Autodesk Inventor part; units mm, degrees
ref_plane "YZ Plane" through (0, 0, 0) normal (1, 0, 0) x (0, 1, 0)
ref_plane "XZ Plane" through (0, 0, 0) normal (0, 1, 0) x (-1, 0, 0)
ref_plane "XY Plane" through (0, 0, 0) normal (0, 0, 1) x (1, 0, 0)
sketch "Sketch1" plane through (0, 0, 0) normal (0, 0, 1) x (1, 0, 0)
  circle A0 centre (0, 0) radius 11
  dimension "d0" = 22
extrude "Extrusion1" add sketch "Sketch1" along normal blind 14
fillet "Fillet1" radius 2 1 edges at (-11, 0, 14)
fillet "Fillet1" radius 4 1 edges at (-11, 0, 0)
hole "Hole1" at (0, 0, 14) direction (0, 0, -1) diameter 13.376 end through all
properties part number "HANDLE CAP" material "Steel, Mild"
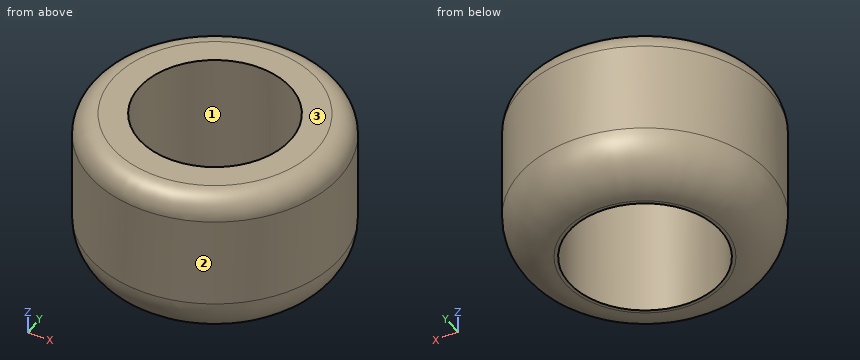
Work out the finished part from the listing and answer in its coordinate system (mm). Face numbers are marked on the shaded views. Round coordinates to 2 decimals unless told otherwise and drop trailing zeros. Write each loop counter-clockwise with the first axis right and the second up, starting at its lowest first coordinate (ties: lowest second). Pieces come first, ordered by that corner, then holes.
1) Consider probe 1 along Y at (x, z) = (0, 6.75); probe 2 along Y at (x, z) = (5.75, 7.75); probe 3 along X at (y, z) = (-2.75, 10.25). Determine where each line is inside the solid, lowest interval first.
2) A cutting plane is placed at C-C on z = 8. Determine the outline of the cut face in (x, y), and give its area (3 significant figures).
3) Determine the mould class of the marked faces 1, 2 and 3 for opening direction Y: pulls with the +Y half, pulls with the -Y half, needs draft (parallel to the pull), parting line crosses it, or undercut.
4) A cutting plane is placed at D-D on z = 3.5. Determine the outline of the cut face in (x, y).
5) Flat-ended cylindrical pins translate along their axes: P1, Ø8, axis at y = -5.5, z = 8, coming from the +X side; P2, Ø4, axis at x = -1, z = 6, coming from the -Y side; P3, Ø6, axis at y = 7, z = 9.5, coming from the -X side; P4, Ø6, axis at y = 5, z = 2, coming from the -X side. Find the tip coordinate at first contact, or state that the pin passes through.
6) A cutting plane is placed at A-A on y = 0. Determine the outline of the cut face in (x, z), and give its area (3 significant figures).
Entries:
1. probe 1: y = -11 to -6.69, 6.69 to 11
1. probe 2: y = -9.38 to -3.42, 3.42 to 9.38
1. probe 3: x = -10.65 to -6.1, 6.1 to 10.65
2. outline: circle Ø22 at (0, 0); hole circle Ø13.38 at (0, 0)
2. area: 240 mm2
3. face 1: undercut
3. face 2: parting line crosses it
3. face 3: needs draft
4. outline: circle Ø21.94 at (0, 0); hole circle Ø13.38 at (0, 0)
5. P1: stops at x = 10.9
5. P2: stops at y = -11
5. P3: stops at x = -10.25
5. P4: stops at x = -10.7
6. outline: (-11, 4) arc R4 ccw to (-7, 0) - (-6.69, 0) - (-6.69, 14) - (-9, 14) arc R2 ccw to (-11, 12) - close; (6.69, 0) - (7, 0) arc R4 ccw to (11, 4) - (11, 12) arc R2 ccw to (9, 14) - (6.69, 14) - close
6. area: 112 mm2
